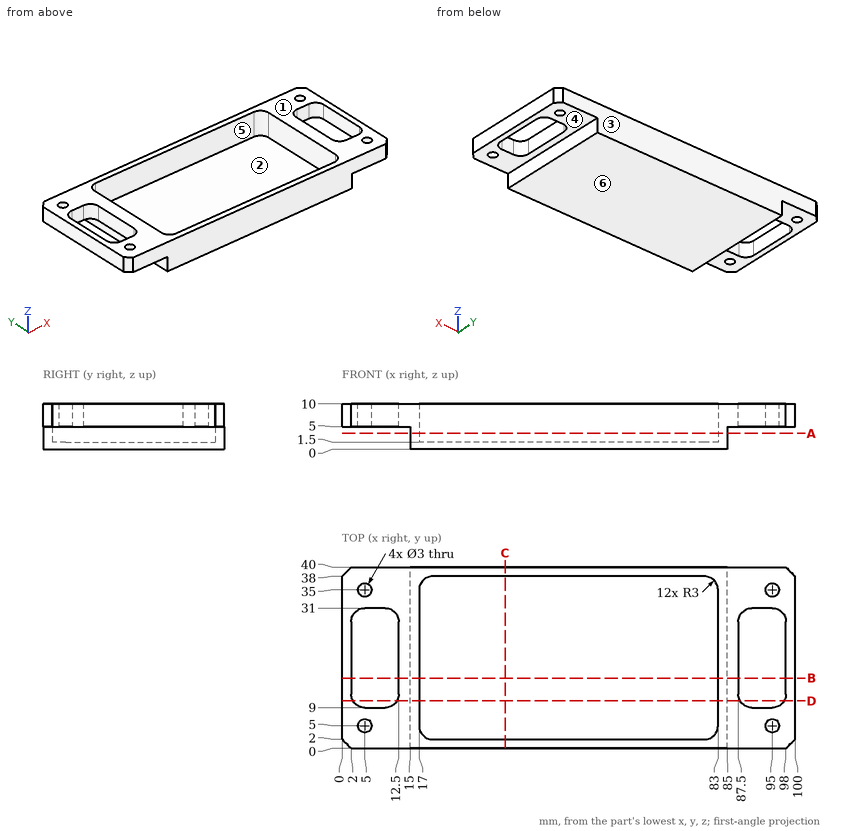
Geometry check sheet. Reference: drawing and pictorial views, mm from the part's lowest x, y, z. A direction names the side the tool comes from. Give positions to 0.01 mm unless a question says otherwise; leave off trailing zeros. Loops run counter-clockwise (first coordinate to the right, second up) from the corner with the lowest first, then second, coordinate; pieces in that order, holes last.
1. Set-up check for the marked faces 4, 5 and 6: record each of +Z, -Z, +X, -X, +Y, -Y from which the full face is reachable in a straight line by a thin tool's end or side.
2. Mould release check, pull along Y, two halves, no side actions. Record for the marked faces 1, 2 and 3: released by +Y, released by -Y, zero draft, split by the parting line, or undercut.
3. Section check C-C, the plane x = 36. Enter the section's corners in (y, z).
4. Thickness scan on line 1 (X direction, y = 23, z = 7.75); line 2 (Y direction, x = 5, z = 8.1); line 3 (X direction, y = 33, z = 2.25). Record the ranges inside material, lowest first.
5. Go/stop test with flat-tipped pins: pin 1 Ø1.5 at (y, z) = (24, 1.5) entering from +X; pin 2 Ø3 at (y, z) = (25.5, 2.5) entering from -X; pin 3 Ø10 at (x, y) = (33.5, 15) entering from +Z. Record where each tip stops, or that it passes through.
6. Section check D-D, the plane y = 10.5. Enter the section's corners in (x, z), then the cut area to 3 significant figures.
7. Section check B-B, the plane y = 15.5. Enter the section's corners in (x, z).
8. Section check A-A, the plane z = 3.5. Enter the section's corners in (x, y), then the cut area to 3 significant figures.
Geometry says:
1. face 4: -Z, +X, +Y, -Y
1. face 5: +Z
1. face 6: -Z, +X, -X, +Y, -Y
2. face 1: zero draft
2. face 2: undercut
2. face 3: released by +Y
3. outline: (0, 0) - (40, 0) - (40, 10) - (38, 10) - (38, 1.5) - (2, 1.5) - (2, 10) - (0, 10) - close
4. line 1: x = 0 to 2, 12.5 to 17, 83 to 87.5, 98 to 100
4. line 2: y = 0 to 3.5, 6.5 to 9, 31 to 33.5, 36.5 to 40
4. line 3: x = 15 to 17, 83 to 85
5. pin 1: stops at x = 85
5. pin 2: stops at x = 15
5. pin 3: stops at z = 1.5
6. outline: (0, 5) - (2.4, 5) - (2.4, 10) - (0, 10) - close; (12.1, 5) - (15, 5) - (15, 0) - (85, 0) - (85, 5) - (87.9, 5) - (87.9, 10) - (83, 10) - (83, 1.5) - (17, 1.5) - (17, 10) - (12.1, 10) - close; (97.6, 5) - (100, 5) - (100, 10) - (97.6, 10) - close
6. area: 192 mm2
7. outline: (0, 5) - (2, 5) - (2, 10) - (0, 10) - close; (12.5, 5) - (15, 5) - (15, 0) - (85, 0) - (85, 5) - (87.5, 5) - (87.5, 10) - (83, 10) - (83, 1.5) - (17, 1.5) - (17, 10) - (12.5, 10) - close; (98, 5) - (100, 5) - (100, 10) - (98, 10) - close
8. outline: (15, 0) - (85, 0) - (85, 40) - (15, 40) - close; hole (17, 5) arc R3 ccw to (20, 2) - (80, 2) arc R3 ccw to (83, 5) - (83, 35) arc R3 ccw to (80, 38) - (20, 38) arc R3 ccw to (17, 35) - close
8. area: 432 mm2
